Read the model definition and answer for the solid it produces. Units are mm, in the model's axes. A direction names the side the tool comes from. Coordinates: 2 decimals unless noted, no trailing zeros. Loops run counter-clockwise (first coordinate to the right, second up) from the corner with the lowest first, then second, coordinate; pieces in that order, holes last. Notation, with made-up numbers: (45.25, -36.75) -> (86.25, -36.75) arc R33 ccw to (86.25, -0.75) -> close; hole circle Ø9 at (14, 55). An arc over 180 degrees is marked (long way). Answer as a JSON object with one key per item and string values. Group by question number.
Q1. Each of these flat-tipped pins is pushed along its axis until it touches: P1, Ø1, axis at y = 8, z = -5, coming from the +X side; P2, Ø1.5, axis at x = 10.5, z = 2, coming from the +Y side; P3, Ø4, axis at x = 5.5, z = 0, coming from the -Y side; P4, Ø9, axis at x = 0, y = 0, coming from the +Z side. Where does it stop, or does it pass through?
Q2. The part is cut by section D-D on y = 9. Write down the section's boundary in (x, z), and give its area (3 significant figures).
Q3. The part is cut by section C-C on z = 3.5. Write down the section's boundary in (x, y), and give its area (3 significant figures).
Q4. For faces 1 (the flat face through (6, 14, 5)), 2 (the flat face through (-4, 4, 6)), determine the directions among +Z, -Z, +X, -X, +Y, -Y from which every point of the face is accessible in a straight line to the end or side of a thin tool.
Q5. Determine the mould class of faces 3 (the flat face through (4, 4, -6)), 4 (the cylindrical face through (-1.08, -4.88, -0.08)), 5 (the cylindrical face through (-2.213, -16.855, -5.507)) for opening direction X: released by +X, released by -X, zero draft, split by the parting line, or undercut.
Q6. The part is cut by section A-A on y = 0. Write down the section's boundary in (x, z), and give its area (3 significant figures).
Q7. Straight lines are drawn through the part: line 1 along Y through (x, z) = (0, 3); line 2 along Z through (x, y) = (15.5, 1); line 3 along Y through (x, z) = (-2, 5.25). For each, find the intervals that lie inside material, in ascending order. Write a range as [from, to].
from build123d import *

# Parameters (mm, degrees)
CUT_EXTRUDE1_DEPTH      = 25.779023387
CUT_EXTRUDE1_DEPTH_BACK = 25.779023387
SKETCH3_R               = 5


with BuildPart() as part:
    # Sketch1 → Revolve1 (revolve)
    with BuildSketch(Plane(origin=(0, 0, 0), x_dir=(0, 0, -1), z_dir=(1, 0, 0)), mode=Mode.PRIVATE) as revolve1_sk:
        Polygon((-5, 17), (-5, 15), (5, 15), (5, 17), (6, 17), (6, 0), (-6, 0), (-6, 17), align=None)
    revolve(revolve1_sk.sketch.rotate(Axis((0, 0, 6), (0, 0, -1)), 90), axis=Axis((0, 0, 6), (0, 0, -1)))

    # Sketch3 → Cut-Extrude1 (cut, two sides: drawn at the far end of the back side and taken through both)
    with BuildSketch(Plane.XY.offset(-CUT_EXTRUDE1_DEPTH_BACK)):
        Circle(SKETCH3_R)
    extrude(amount=CUT_EXTRUDE1_DEPTH + CUT_EXTRUDE1_DEPTH_BACK, mode=Mode.SUBTRACT)


solid = part.part
Final values:
{
 "1": {"P1": "stops at x = 15.26", "P2": "stops at y = 11.4", "P3": "stops at y = -14.59", "P4": "passes through"},
 "2": {"outline": "(-14.42, -6) -> (14.42, -6) -> (14.42, -5) -> (12, -5) -> (12, 5) -> (14.42, 5) -> (14.42, 6) -> (-14.42, 6) -> (-14.42, 5) -> (-12, 5) -> (-12, -5) -> (-14.42, -5) -> close", "area": "298 mm2"},
 "3": {"outline": "circle Ø30 at (0, 0); hole circle Ø10 at (0, 0)", "area": "628 mm2"},
 "4": {"face 1": "none", "face 2": "+Z, +X, -X, +Y, -Y"},
 "5": {"face 3": "zero draft", "face 4": "undercut", "face 5": "split by the parting line"},
 "6": {"outline": "(-17, -6) -> (-5, -6) -> (-5, 6) -> (-17, 6) -> (-17, 5) -> (-15, 5) -> (-15, -5) -> (-17, -5) -> close; (5, -6) -> (17, -6) -> (17, -5) -> (15, -5) -> (15, 5) -> (17, 5) -> (17, 6) -> (5, 6) -> close", "area": "248 mm2"},
 "7": {"line 1": "y = [-15, -5], [5, 15]", "line 2": "z = [-6, -5], [5, 6]", "line 3": "y = [-16.88, -4.58], [4.58, 16.88]"}
}
